The listing builds one solid part. Answer for the finished solid, in the listing's coordinates (mm). Face numbers are marked on the shaded views. A direction names the side the tool comes from. Coordinates: 2 decimals unless noted, no trailing zeros. Write each loop counter-clockwise with the first axis right and the second up, starting at its lowest first coordinate (ties: lowest second). Pieces come first, ordered by that corner, then holes.
from build123d import *

# Parameters (mm, degrees)
F0_W     = 30
F0_H     = 25
F1_DEPTH = 25.4
F2_SIZE  = 5.08
F3_W     = 13.087139
F3_H     = 10.707659
F4_DEPTH = 35.941


with BuildPart() as f1:
    # F0 (on Top) → F1 (new body)
    with BuildSketch(Plane.XY):
        with Locations((9.369201, 1.240393)):
            Rectangle(F0_W, F0_H)
    extrude(amount=F1_DEPTH)

    # F2
    f2_edges = [f1.edges().sort_by_distance(p)[0] for p in [
        (24.369201, -11.259607, 12.7),
    ]]
    chamfer(f2_edges, length=F2_SIZE)

    # F3 (on face) → F4 (cut)
    with BuildSketch(Plane.XZ.offset(11.259607)):
        with Locations((6.543569, 11.302529)):
            Rectangle(F3_W, F3_H)
    extrude(amount=-F4_DEPTH, mode=Mode.SUBTRACT)


solid = f1.part
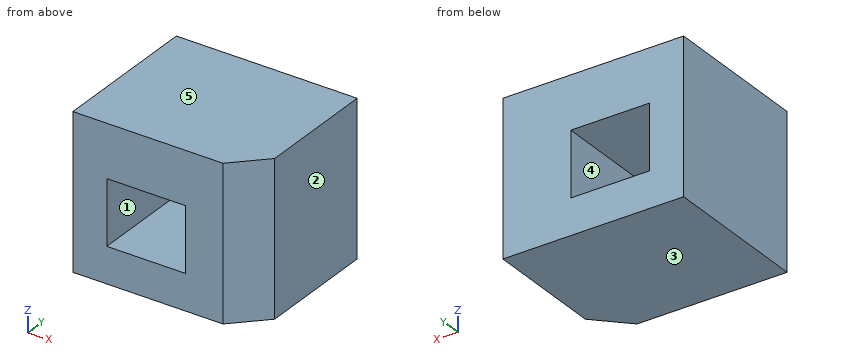
1. For a pull along Z with two mould halves and no side action, classify the marked faces 1, 2 and 3 as pulls with the +Z half, pulls with the -Z half, needs draft (parallel to the pull), parting line crosses it, or undercut.
Results found:
face 1: undercut
face 2: needs draft
face 3: pulls with the -Z half
2. Section B-B on y = -1.25 is taken. Give the vertices of the cut face in (x, z).
Results found:
outline: (-5.63, 0) - (24.37, 0) - (24.37, 25.4) - (-5.63, 25.4) - close; hole (0, 5.95) - (13.09, 5.95) - (13.09, 16.66) - (0, 16.66) - close
3. Section C-C on z = 14.75 is taken. Give the vertices of the cut face in (x, y).
Results found:
outline: (-5.63, -11.26) - (0, -11.26) - (0, 13.74) - (-5.63, 13.74) - close; (13.09, -11.26) - (19.29, -11.26) - (24.37, -6.18) - (24.37, 13.74) - (13.09, 13.74) - close
4. A tool of negligible diameter and unlimited length cuts with its end or side. For the marked faces 4 and 5, from which of +Z, -Z, +X, -X, +Y, -Y can it reach the whole face along a straight path? Write none if from no direction.
Results found:
face 4: +Y, -Y
face 5: +Z, +X, -X, +Y, -Y
5. Section D-D on z = 3.25 is taken. Give the vertices of the cut face in (x, y), then the cut area to 3 significant figures.
Results found:
outline: (-5.63, -11.26) - (19.29, -11.26) - (24.37, -6.18) - (24.37, 13.74) - (-5.63, 13.74) - close
area: 737 mm2
6. A flat-ended cylindrical pin translates along its axis: P1, Ø3, axis at x = 5.5, z = 8, coming from the -Y side. Find the tip coordinate at first contact, or state that the pin passes through.
Results found:
P1: passes through
7. Section A-A on x = 12 is taken. Give the vertices of the cut face in (y, z), then the cut area to 3 significant figures.
Results found:
outline: (-11.26, 0) - (13.74, 0) - (13.74, 5.95) - (-11.26, 5.95) - close; (-11.26, 16.66) - (13.74, 16.66) - (13.74, 25.4) - (-11.26, 25.4) - close
area: 367 mm2
8. Find the intervals of material crossed by L1, parallel to Z at x = 1, y = 1; L2, parallel to X at y = 3.25, z = 12.5; L3, parallel to X at y = -8.25, z = 10, in increasing order.
Results found:
L1: z = 0 to 5.95, 16.66 to 25.4
L2: x = -5.63 to 0, 13.09 to 24.37
L3: x = -5.63 to 0, 13.09 to 22.3
